Geometry check sheet. Reference: the model listing, model coordinates, mm. A direction names the side the tool comes from. Give positions to 0.01 mm unless a question says otherwise; leave off trailing zeros. Loops run counter-clockwise (first coordinate to the right, second up) from the corner with the lowest first, then second, coordinate; pieces in that order, holes last. Notation, with made-up numbers: (52, 52.5) - (110, 52.5) arc R12 ccw to (110, 75.5) - close; hole circle Ø9 at (19.25, 10.5). An arc over 180 degrees is marked (long way). Use a Markdown table: item, result. Add a question column.
1. Cross-section at D-D on x = -10. Enter the section's corners in (y, z), and give its area (3 significant figures).
2. Depth check by flat-ended pin: P1, Ø3, axis at x = 11, z = 9.5, coming from the +Y side; P2, Ø2, axis at x = -10, y = 34, coming from the +Z side; P3, Ø8, axis at x = 4.5, y = 33.5, coming from the +Z side; P4, Ø6, axis at x = -10, z = 8.5, coming from the -Y side. Enter the tip coordinate at first touch or a pass-through.
3. Cross-section at A-A on x = 10. Enter the section's corners in (y, z), and give its area (3 significant figures).
4. Set-up check for faces 1 (the flat face through (0, 25, 10)), 2 (the cylindrical face through (7.95, 3.65, 16.48)), 3 (the flat face through (0, 0, 16)), 4 (the flat face through (0, 34, 6)): record each of +Z, -Z, +X, -X, +Y, -Y from which the full face is reachable in a straight line by a thin tool's end or side.
5. Material ranges on L1, parallel to Z at x = -11.5, y = 15; L2, parallel to Y at x = -10, z = 4.15; L3, parallel to Y at x = 11, z = 9.75, recorded low to high.
6. Cross-section at C-C on y = 3. Enter the section's corners in (x, z).
7. Cross-section at B-B on y = 16.5. Enter the section's corners in (x, z).
8. Draft check along Z on faces 5 (the flat face through (0, 20, 0)), 6 (the flat face through (-14, 20, 3)), 7 (the flat face through (0, 13, 15)). Enter one of: pulls with the +Z half, pulls with the -Z half, needs draft (parallel to the pull), parting line crosses it, or undercut.
from build123d import *

# Parameters (mm, degrees)
EXTRUDE_1_DEPTH          = 14
HOLE_WIZARD_M4_1_D       = 3.3
HOLE_WIZARD_M4_2_D       = 3.3
HOLE_WIZARD_M4_2_DEPTH   = 5
HOLE_WIZARD_M4_1_2_D     = 4.3
HOLE_WIZARD_M4_1_2_DEPTH = 3


with BuildPart() as part:
    # 草图2 → 凸台-拉伸1 (new, symmetric)
    with BuildSketch(Plane(origin=(0, 0, 0), x_dir=(0, 0, -1), z_dir=(1, 0, 0))):
        Polygon((-15, 0), (-18, 0), (-18, 29), (-6, 29), (-6, 39), (0, 39), (0, 0), (-5, 0), (-5, 25), (-15, 25), align=None)
    extrude(amount=EXTRUDE_1_DEPTH, both=True)

    # Hole Wizard M4 _1 (through all)
    with Locations(Plane.XY.offset(6)):
        with Locations((-10, 34)):
            Hole(HOLE_WIZARD_M4_1_D / 2)

    # M4 螺纹孔2
    with Locations(Plane(origin=(0, 0, 0), x_dir=(-1, 0, 0), z_dir=(0, 0, -1))):
        with Locations((10, 3), (-10, 3)):
            Hole(HOLE_WIZARD_M4_2_D / 2, depth=HOLE_WIZARD_M4_2_DEPTH)

    # Hole Wizard M4 _1 2
    with Locations(Plane.XY.offset(18)):
        with Locations((-10, 3), (10, 3)):
            Hole(HOLE_WIZARD_M4_1_2_D / 2, depth=HOLE_WIZARD_M4_1_2_DEPTH)


solid = part.part
Values found:
| question | item | result |
|---|---|---|
| 1 | outline | (0, 0) - (1.35, 0) - (1.35, 5) - (0, 5) - close; (0, 15) - (0.85, 15) - (0.85, 18) - (0, 18) - close; (4.65, 0) - (32.35, 0) - (32.35, 6) - (29, 6) - (29, 18) - (5.15, 18) - (5.15, 15) - (25, 15) - (25, 5) - (4.65, 5) - close; (35.65, 0) - (39, 0) - (39, 6) - (35.65, 6) - close |
| 1 | area | 283 mm2 |
| 2 | P1 | stops at y = 29 |
| 2 | P2 | passes through |
| 2 | P3 | stops at z = 6 |
| 2 | P4 | stops at y = 25 |
| 3 | outline | (0, 0) - (1.35, 0) - (1.35, 5) - (0, 5) - close; (0, 15) - (0.85, 15) - (0.85, 18) - (0, 18) - close; (4.65, 0) - (39, 0) - (39, 6) - (29, 6) - (29, 18) - (5.15, 18) - (5.15, 15) - (25, 15) - (25, 5) - (4.65, 5) - close |
| 3 | area | 303 mm2 |
| 4 | face 1 | +X, -X, -Y |
| 4 | face 2 | +Z |
| 4 | face 3 | +Z, -Z, +X, -X, -Y |
| 4 | face 4 | +Z, +X, -X, +Y |
| 5 | L1 | z = 0 to 5, 15 to 18 |
| 5 | L2 | y = 0 to 1.35, 4.65 to 32.35, 35.65 to 39 |
| 5 | L3 | y = 25 to 29 |
| 6 | outline | (-14, 0) - (-11.65, 0) - (-11.65, 5) - (-14, 5) - close; (-14, 15) - (-12.15, 15) - (-12.15, 18) - (-14, 18) - close; (-8.35, 0) - (8.35, 0) - (8.35, 5) - (-8.35, 5) - close; (-7.85, 15) - (7.85, 15) - (7.85, 18) - (-7.85, 18) - close; (11.65, 0) - (14, 0) - (14, 5) - (11.65, 5) - close; (12.15, 15) - (14, 15) - (14, 18) - (12.15, 18) - close |
| 7 | outline | (-14, 0) - (14, 0) - (14, 5) - (-14, 5) - close; (-14, 15) - (14, 15) - (14, 18) - (-14, 18) - close |
| 8 | face 5 | pulls with the -Z half |
| 8 | face 6 | needs draft |
| 8 | face 7 | undercut |
